from build123d import *

# Parameters (mm, degrees)
BOSS_EXTRUDE1_DEPTH      = 10
CHAMFER1_SIZE            = 3
BOSS_EXTRUDE2_START      = -1.5
BOSS_EXTRUDE2_DEPTH      = 1.5
CHAMFER1_OF_MIRROR1_SIZE = 3
SKETCH2_W                = 16
SKETCH2_H                = 8.5
CUT_EXTRUDE1_DEPTH       = 39.340066647
CHAMFER2_SIZE            = 1.25


with BuildPart() as part:
    # Sketch1 → Boss-Extrude1 (new body)
    # profile 1 of 2: a face of its own
    with BuildSketch(Plane.XY):
        Polygon((30, 5.5), (30, -5.5), (0, -6.5), (0, 6.5), align=None)
        with BuildLine():
            ThreePointArc((5, 4), (1, 0), (5, -4))
            Line((5, -4), (25, -4))
            ThreePointArc((25, -4), (29, 0), (25, 4))
            Line((25, 4), (5, 4))
        make_face(mode=Mode.SUBTRACT)
    # profile 2 of 2: a face of its own
    with BuildSketch(Plane.XY):
        with BuildLine():
            Line((5, 4), (25, 4))
            ThreePointArc((25, 4), (29, 0), (25, -4))
            Line((25, -4), (5, -4))
            ThreePointArc((5, -4), (1, 0), (5, 4))
        make_face()
        with BuildLine():
            ThreePointArc((25, -3), (28, 0), (25, 3))
            Line((25, 3), (5, 3))
            ThreePointArc((5, 3), (2, 0), (5, -3))
            Line((5, -3), (25, -3))
        make_face(mode=Mode.SUBTRACT)
    boss_extrude1 = extrude(amount=BOSS_EXTRUDE1_DEPTH)

    # Chamfer1
    chamfer1_edges = [part.edges().sort_by_distance(p)[0] for p in [
        (30, -5.5, 5),
        (0, -6.5, 5),
        (0, 6.5, 5),
        (30, 5.5, 5),
    ]]
    chamfer(chamfer1_edges, length=CHAMFER1_SIZE)

    # Sketch1<4> → Boss-Extrude2 (add)
    with BuildSketch(Plane.XY.offset(BOSS_EXTRUDE2_START)):
        with BuildLine():
            Line((5, 4), (25, 4))
            ThreePointArc((25, 4), (29, 0), (25, -4))
            Line((25, -4), (5, -4))
            ThreePointArc((5, -4), (1, 0), (5, 4))
        make_face()
        with BuildLine():
            ThreePointArc((25, -3), (28, 0), (25, 3))
            Line((25, 3), (5, 3))
            ThreePointArc((5, 3), (2, 0), (5, -3))
            Line((5, -3), (25, -3))
        make_face(mode=Mode.SUBTRACT)
    boss_extrude2 = extrude(amount=BOSS_EXTRUDE2_DEPTH)


with BuildPart() as mirror1_1:
    # Mirror1: Boss-Extrude1, Boss-Extrude2 across plane
    add(boss_extrude1.mirror(Plane.XY.offset(10)))
    add(boss_extrude2.mirror(Plane.XY.offset(10)))

    # Chamfer1 of Mirror1
    chamfer1_of_mirror1_edges = [mirror1_1.edges().sort_by_distance(p)[0] for p in [
        (30, -5.5, 15),
        (0, -6.5, 15),
        (0, 6.5, 15),
        (30, 5.5, 15),
    ]]
    chamfer(chamfer1_of_mirror1_edges, length=CHAMFER1_OF_MIRROR1_SIZE)


with BuildPart() as part_1:
    add(part.part)

    # Mirror1 united with what the copies touc: union Mirror1_1
    add(mirror1_1.part)

    # Sketch2 → Cut-Extrude1 (cut, through all)
    with BuildSketch(Plane.XY.offset(21.5)):
        with Locations((15, 0)):
            Rectangle(SKETCH2_W, SKETCH2_H)
    extrude(amount=-CUT_EXTRUDE1_DEPTH, mode=Mode.SUBTRACT)

    # Chamfer2
    chamfer2_edges = [part_1.edges().sort_by_distance(p)[0] for p in [
        (23, -3, 10),
        (23, 3, 10),
        (7, -3, 10),
        (7, 3, 10),
    ]]
    chamfer(chamfer2_edges, length=CHAMFER2_SIZE - 0.0001)  # a hair under: the kernel refuses the full size


solid = part_1.part
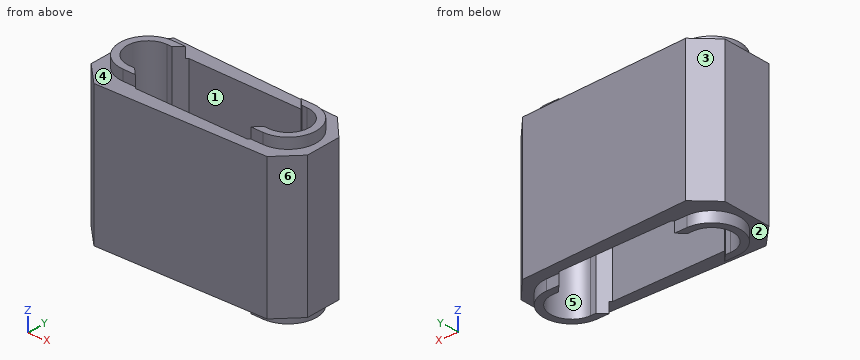
Here's how the part is built. I have some questions about the finished solid (model axes, mm). Face numbers are marked on the shaded views. A direction names the side the tool comes from. Round coordinates to 2 decimals unless told otherwise and drop trailing zeros. Write each loop counter-clockwise with the first axis right and the second up, starting at its lowest first coordinate (ties: lowest second). Pieces come first, ordered by that corner, then holes.
1. For the marked faces 4, 5 and 6, which set-ups out of +Z, -Z, +X, -X, +Y, -Y let a thin tool reach every point of the face, with its end or its side?
2. If we mould it in two halves opening along Y, with no side actions, what happens to the marked faces 1, 2 and 3? For each: released by +Y, released by -Y, zero draft, split by the parting line, or undercut.
3. I need wall thicknesses on L1, parallel to Z at x = 2.5, y = 4.5; L2, parallel to X at y = 3.25, z = 18.25; L3, parallel to Y at x = 14, z = 18.25. Which ranges of each line are inside material? Lowest first, please.
4. Suppose I cut it at D-D (y = 1.5). List the corners of the cut face in (x, z) for me.
5. Suppose I cut it at C-C (x = 21). List the corners of the cut face in (y, z) for me.
6. Will these pins go through, and if not, where does the flat tip stop? pin 1 Ø4 at (x, y) = (13.5, -2) entering from -Z; pin 2 Ø0.8 at (x, z) = (24.5, 12.5) entering from +Y; pin 3 Ø4 at (x, z) = (18, 10) entering from +Y; pin 4 Ø0.8 at (x, z) = (24, -0.5) entering from +Y.
7. Suppose I cut it at A-A (y = 0). List the corners of the cut face in (x, z) for me.
Answer sheet:
1. face 4: +Z
1. face 5: +Z, -Z
1. face 6: +Z, -Z, +X, -Y
2. face 1: undercut
2. face 2: zero draft
2. face 3: released by +Y
3. L1: z = 0 to 20
3. L2: x = 0 to 6, 24 to 29.27
3. L3: y = -6.03 to -4.25, 4.25 to 6.03
4. outline: (0, 0) - (1.29, 0) - (1.29, -1.5) - (2.4, -1.5) - (2.4, 21.5) - (1.29, 21.5) - (1.29, 20) - (0, 20) - close; (27.6, -1.5) - (28.71, -1.5) - (28.71, 0) - (30, 0) - (30, 20) - (28.71, 20) - (28.71, 21.5) - (27.6, 21.5) - close
5. outline: (-5.8, 0) - (-4.25, 0) - (-4.25, 20) - (-5.8, 20) - close; (4.25, 0) - (5.8, 0) - (5.8, 20) - (4.25, 20) - close
6. pin 1: passes through
6. pin 2: stops at y = 5.7
6. pin 3: stops at y = 5.97
6. pin 4: stops at y = 4
7. outline: (0, 0) - (1, 0) - (1, -1.5) - (2, -1.5) - (2, 21.5) - (1, 21.5) - (1, 20) - (0, 20) - close; (28, -1.5) - (29, -1.5) - (29, 0) - (30, 0) - (30, 20) - (29, 20) - (29, 21.5) - (28, 21.5) - close
